Could you check a few things on this model? Use its own coordinates, in mm. A direction names the side the tool comes from. Coordinates: 2 decimals unless noted, no trailing zeros. Order: outer loops, then holes, each group sorted by start corner. A loop starts at its lowest first (then second) coordinate and runs counter-clockwise, first axis right, second up.
```python
from build123d import *

# Parameters (mm, degrees)
F0_W     = 112.308848
F0_H     = 25.530828
F1_DEPTH = 88.9
F2_R     = 20.581967
F3_DEPTH = 25.4
F5_DEPTH = 177.8


with BuildPart() as f1:
    # F0 (on Front) → F1 (new body)
    with BuildSketch(Plane.XZ):
        with Locations((-18.293744, -12.765414)):
            Rectangle(F0_W, F0_H)
    extrude(amount=-F1_DEPTH)

    # F2 (on Top) → F3 (join)
    with BuildSketch(Plane.XY):
        with Locations((-19.09228, 44.607155)):
            Circle(F2_R)
    extrude(amount=F3_DEPTH)

    # F4 (on Front) → F5 (cut)
    with BuildSketch(Plane.XZ):
        Polygon((5.159772, 39.870981), (-63.458517, 37.190579), (5.159772, 3.149472), align=None)
    extrude(amount=-F5_DEPTH, mode=Mode.SUBTRACT)


solid = f1.part
```
Item 1: Suppose I cut it at A-A (y = 34). List the corners of the cut face in (x, z) for me, and give its area (3 significant figures).
Item 2: Suppose I cut it at B-B (x = -55). List the corners of the cut face in (y, z) for me.
Item 3: Suppose I cut it at D-D (x = -24). List the corners of the cut face in (y, z) for me, and give its area (3 significant figures).
Item 4: Suppose I cut it at C-C (z = 19). List the corners of the cut face in (x, y) for me.
Item 5: I need wall thicknesses on line 1 (Z direction, x = 19.5, y = 37); line 2 (Z direction, x = -12, y = 29.5); line 3 (Y direction, x = -33, z = 13). Which ranges of each line are inside material? Lowest first, please.
Item 6: Which directions (+Z, -Z, +X, -X, +Y, -Y) give clear straight access to the entire face, cutting with the end or side of a thin tool? Please do faces 1 (the face through (-39.654, 45.512, 9.858)), 2 (the face through (-19, 0, -13)).
Item 7: For pin 1 Ø3 at (x, y) = (-42, 17.5) entering from +Z; pin 2 Ø12 at (y, z) = (42.5, 15) entering from -X; pin 3 Ø10 at (x, y) = (-28, 59.5) entering from +Z, each with a flat end and sliding along its axis, tell me the tip position at first contact or that it passes through.
Geometry results:
1. outline: (-74.45, -25.53) - (37.86, -25.53) - (37.86, 0) - (-1.45, 0) - (-1.45, 6.43) - (-36.73, 23.93) - (-36.73, 0) - (-74.45, 0) - close
1. area: 3,400 mm2
2. outline: (0, -25.53) - (88.9, -25.53) - (88.9, 0) - (0, 0) - close
3. outline: (0, -25.53) - (88.9, -25.53) - (88.9, 0) - (64.6, 0) - (64.6, 17.62) - (24.62, 17.62) - (24.62, 0) - (0, 0) - close
3. area: 2,970 mm2
4. outline: (-26.79, 25.52) - (-26.79, 63.7) arc R20.58 ccw to start
5. line 1: z = -25.53 to 0
5. line 2: z = -25.53 to 11.66
5. line 3: y = 29.44 to 59.78
6. face 1: +Z
6. face 2: +Z, -Z, +X, -X, -Y
7. pin 1: stops at z = 0
7. pin 2: stops at x = -39.67
7. pin 3: stops at z = 22.08
